The model under review builds one solid part; all positions refer to its coordinate system, in mm. Face numbers are marked on the shaded views. Coordinates: 2 decimals unless noted, no trailing zeros. Order: outer loops, then holes, each group sorted by start corner. A loop starts at its lowest first (then second) coordinate and runs counter-clockwise, first axis right, second up. Notation, with made-up numbers: (-36, 63) - (23, 63) arc R23 ccw to (23, 102) - close; hole circle Ø2 at (81, 69). An arc over 180 degrees is marked (long way). Answer in a Markdown table with one row per item.
```python
from build123d import *

# Parameters (mm, degrees)
EXTRUDE_1_DEPTH     = 75
SHELL_1_T           = -5
SKETCH_2_W          = 65
SKETCH_2_H          = 5
CUT_EXTRUDE_1_DEPTH = 25
SKETCH_3_R          = 3.25
CUT_EXTRUDE_2_DEPTH = 21
SKETCH_4_W          = 30
SKETCH_4_H          = 5
EXTRUDE_2_DEPTH     = 10
EXTRUDE_3_DEPTH     = 75
SKETCH_8_R          = 2
CUT_EXTRUDE_4_DEPTH = 6
CUT_EXTRUDE_5_DEPTH = 3


with BuildPart() as part:
    # 草图1 → 凸台-拉伸1 (new body)
    with BuildSketch(Plane.XY):
        Polygon((0, 0), (30, 0), (30, 27.320508076), (0, 10), align=None)
    extrude(amount=EXTRUDE_1_DEPTH)

    # 抽壳1
    shell_1_openings = [part.faces().sort_by_distance(p)[0] for p in [
        (30, 13.660254038, 37.5),
    ]]
    offset(amount=SHELL_1_T, openings=shell_1_openings, kind=Kind.INTERSECTION)

    # 草图2 → 切除-拉伸1 (cut)
    with BuildSketch(Plane(origin=(30, 0, 0), x_dir=(0, 0, -1), z_dir=(1, 0, 0))):
        with Locations((-37.5, 2.5)):
            Rectangle(SKETCH_2_W, SKETCH_2_H)
    extrude(amount=-CUT_EXTRUDE_1_DEPTH, mode=Mode.SUBTRACT)

    # 草图3 → 切除-拉伸2 (cut, through all)
    with BuildSketch(Plane(origin=(-1.830127019, 3.169872981, 0), x_dir=(0.866025404, 0.5, 0), z_dir=(0.5, -0.866025404, 0))):
        with Locations((27.886751346, 37.5)):
            Circle(SKETCH_3_R)
    extrude(amount=-CUT_EXTRUDE_2_DEPTH, mode=Mode.SUBTRACT)

    # 草图4 → 凸台-拉伸2 (add)
    with BuildSketch(Plane.XY.offset(75)):
        with Locations((15, 2.5)):
            Rectangle(SKETCH_4_W, SKETCH_4_H)
    extrude_2 = extrude(amount=EXTRUDE_2_DEPTH)

    # 镜向1: 凸台-拉伸2 across plane
    add(extrude_2.mirror(Plane.XY.offset(37.5)))

    # 草图5 → 凸台-拉伸3 (add)
    with BuildSketch(Plane.XY.offset(75)):
        Polygon((0, 10), (-11.353593044, 3.445), (-9.364621366, 0), (0, 0), align=None)
    extrude(amount=-EXTRUDE_3_DEPTH)

    # 草图8 → 切除-拉伸4 (cut, through all)
    with BuildSketch(Plane(origin=(0, 5, 0), x_dir=(1, 0, 0), z_dir=(0, 1, 0))):
        with Locations((15, 5)):
            Circle(SKETCH_8_R)
    cut_extrude_4 = extrude(amount=-CUT_EXTRUDE_4_DEPTH, mode=Mode.SUBTRACT)

    # 草图9 → 切除-拉伸5 (cut)
    with BuildSketch(Plane(origin=(0, 5, 0), x_dir=(1, 0, 0), z_dir=(0, 1, 0))):
        Polygon((17.020725942, 8.5), (12.979274058, 8.5), (10.958548116, 5), (12.979274058, 1.5), (17.020725942, 1.5), (19.041451884, 5), align=None)
    cut_extrude_5 = extrude(amount=-CUT_EXTRUDE_5_DEPTH, mode=Mode.SUBTRACT)

    # 镜向2: 切除-拉伸4, 切除-拉伸5 across plane
    add(cut_extrude_4.mirror(Plane.XY.offset(37.5)), mode=Mode.SUBTRACT)
    add(cut_extrude_5.mirror(Plane.XY.offset(37.5)), mode=Mode.SUBTRACT)


solid = part.part
```
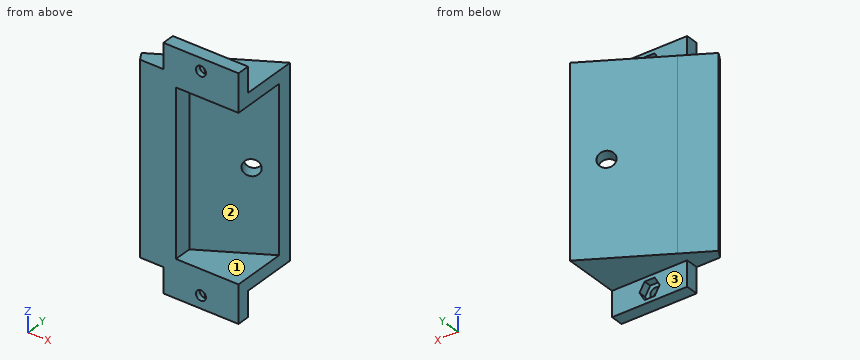
Item 1: Clearance check with flat-ended pins moving along their axes: pin 1 Ø3 at (x, z) = (12, -3.5) entering from +Y; pin 2 Ø10 at (x, z) = (18.5, 35) entering from -Y; pin 3 Ø3 at (y, z) = (22, 28.5) entering from -X. State where each tip first meets the part, or that it passes through.
Check values:
| item | result |
|---|---|
| pin 1 | y = 5 |
| pin 2 | y = 12.02 |
| pin 3 | x = 18.19 |
Item 2: We need section C-C, the plane y = 8. Write out the cut boundary in (x, z).
Check values:
| item | result |
|---|---|
| outline | (-3.46, 0) - (30, 0) - (30, 5) - (6.54, 5) - (6.54, 70) - (30, 70) - (30, 75) - (-3.46, 75) - close |
Item 3: Mouldability with a two-part tool opening along Z and no side actions: class the marked faces 1, 2 and 3 as +Z half, -Z half, draft (parallel to the pull), parting line (faces both ways), or undercut.
Check values:
| item | result |
|---|---|
| face 1 | undercut |
| face 2 | undercut |
| face 3 | draft |
Item 4: We need section D-D, the plane x = 27. Write out the cut boundary in (y, z), then the cut area to 3 significant figures.
Check values:
| item | result |
|---|---|
| outline | (0, -10) - (5, -10) - (5, 0) - (25.59, 0) - (25.59, 75) - (5, 75) - (5, 85) - (0, 85) - (0, 70) - (19.81, 70) - (19.81, 5) - (0, 5) - close |
| area | 731 mm^2 |
Item 5: We need section A-A, the plane x = 15. Write out the cut boundary in (y, z), then the cut area to 3 significant figures.
Check values:
| item | result |
|---|---|
| outline | (0, -10) - (5, -10) - (5, -8.5) - (2, -8.5) - (2, -7) - (0, -7) - close; (0, -3) - (2, -3) - (2, -1.5) - (5, -1.5) - (5, 0) - (18.66, 0) - (18.66, 75) - (5, 75) - (5, 76.5) - (2, 76.5) - (2, 78) - (0, 78) - (0, 70) - (12.89, 70) - (12.89, 5) - (0, 5) - close; (0, 82) - (2, 82) - (2, 83.5) - (5, 83.5) - (5, 85) - (0, 85) - close |
| area | 604 mm^2 |
Item 6: We need section B-B, the plane z = 51.5. Write out the cut boundary in (x, y) (1 decimal), then the cut area to 3 significant figures.
Check values:
| item | result |
|---|---|
| outline | (-11.4, 3.4) - (-9.4, 0) - (5, 0) - (5, 7.1) - (30, 21.5) - (30, 27.3) - close |
| area | 274 mm^2 |
Item 7: To check wall thickness, follow line 1 (Z direction, x = 15, y = 1.5); line 2 (X direction, y = 1.2, z = 80); line 3 (Z direction, x = 22, y = 17.75). State the ranges of each line that lie inside material, in increasing order. Write a range as from..to.
Check values:
| item | result |
|---|---|
| line 1 | -10..-7, -3..5, 70..78, 82..85 |
| line 2 | 0..13, 17..30 |
| line 3 | 0..34.25, 40.75..75 |
